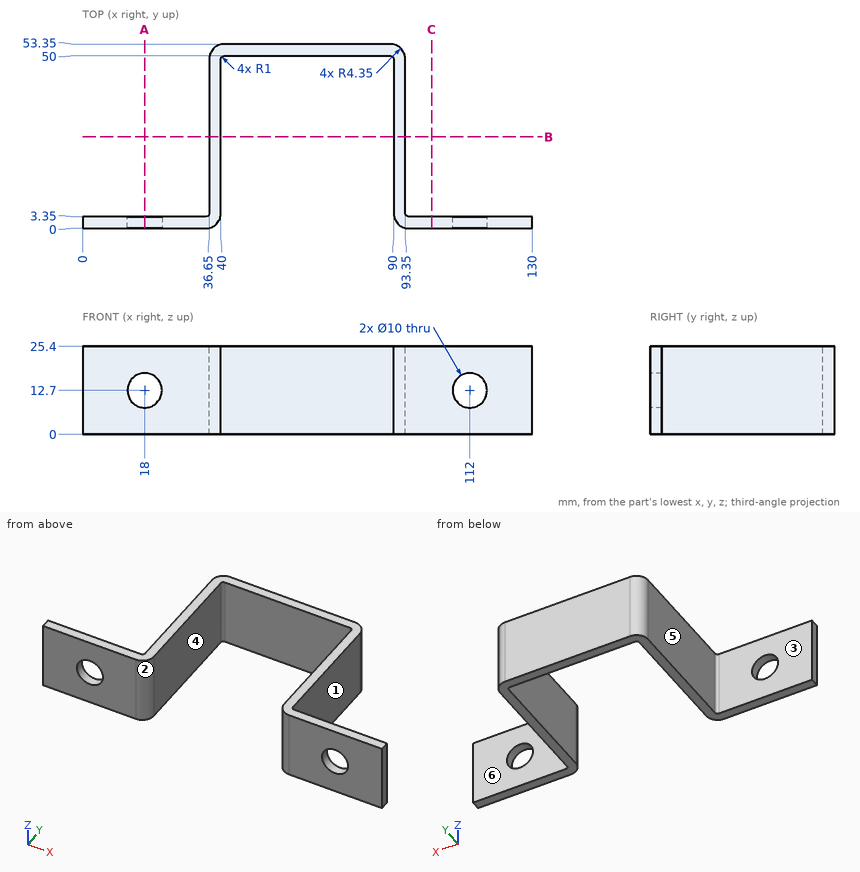
Verification items for this drawing (mm, ordinates from the low corner). A direction names the side the tool comes from. Round coordinates to 2 decimals unless told otherwise and drop trailing zeros. Write each loop counter-clockwise with the first axis right and the second up, starting at its lowest first coordinate (ties: lowest second). Pieces come first, ordered by that corner, then holes. Notation, with made-up numbers: M -38,11.25 L 19,11.25 A14 ccw 19,20.25 Z; hole C -29.75,41 d10. An arc over 180 degrees is marked long. Write item = value, one per line. Start each with the question number.
1. Release check for a two-part mould opening along X. For the marked faces 1, 2 and 3 record: pulls with the +X half, pulls with the -X half, needs draft (parallel to the pull), parting line crosses it, or undercut.
2. Section check B-B, the plane y = 26.5. Record the cut outline in (x, z), then the cut area to 3 significant figures.
3. Scan lines: line 1 (Z direction, x = 18, y = 2.1); line 2 (X direction, y = 41.5, z = 23.5); line 3 (Y direction, x = 41, z = 21.5). Record each from-to range of solid material in increasing order. Write a range as [from, to].
4. Gauge pin test, flat ends, axial feed: pin 1 (8 mm diameter, centred on x = 14, z = 15.5, fed in from -Y); pin 2 (6 mm diameter, centred on x = 86.5, y = 44.5, fed in from -Z); pin 3 (12.5 mm diameter, centred on y = 26.5, z = 7, fed in from +X); pin 4 (12.5 mm diameter, centred on y = 23, z = 9, fed in from -X). Record the tip position at first contact, or that the pin passes through.
5. Section check A-A, the plane x = 18. Record the cut outline in (y, z), then the cut area to 3 significant figures.
6. Section check C-C, the plane x = 101. Record the cut outline in (y, z), then the cut area to 3 significant figures.
7. Tool access check on the marked faces 4, 5 and 6. Record the directions out of +Z, -Z, +X, -X, +Y, -Y that give a thin tool (end or side, any length) a straight path to the whole face; none if there is none.
Results found:
q1.face_1 = pulls with the +X half
q1.face_2 = undercut
q1.face_3 = needs draft
q2.outline = M 36.65,0 L 40,0 L 40,25.4 L 36.65,25.4 Z; M 90,0 L 93.35,0 L 93.35,25.4 L 90,25.4 Z
q2.area = 170 mm^2
q3.line_1 = [0, 7.7], [17.7, 25.4]
q3.line_2 = [36.65, 40], [90, 93.35]
q3.line_3 = [50, 53.35]
q4.pin_1 = 0
q4.pin_2 = through
q4.pin_3 = 93.35
q4.pin_4 = 36.65
q5.outline = M 0,0 L 3.35,0 L 3.35,7.7 L 0,7.7 Z; M 0,17.7 L 3.35,17.7 L 3.35,25.4 L 0,25.4 Z
q5.area = 51.6 mm^2
q6.outline = M 0,0 L 3.35,0 L 3.35,25.4 L 0,25.4 Z
q6.area = 85.1 mm^2
q7.face_4 = +Z, -Z, -Y
q7.face_5 = +Z, -Z, -X, +Y
q7.face_6 = +Z, -Z, +X, +Y
